Read the model definition and answer for the solid it produces. Units are mm, in the model's axes. Face numbers are marked on the shaded views. A direction names the side the tool comes from. Coordinates: 2 decimals unless noted, no trailing zeros. Write each loop counter-clockwise with the first axis right and the second up, starting at its lowest first coordinate (ties: lowest second). Pieces come first, ordered by that corner, then holes. Notation, with made-up numbers: (86.5, 82.5) -> (122.5, 82.5) arc R13 ccw to (122.5, 93.5) -> close; hole circle Ø9 at (36.25, 20). An arc over 180 degrees is marked (long way). Answer as a JSON object with one key per item and string values. Group by question number.
(1) Find section D-D (z = 27). Give the vertices of the cut face in (x, y), then the cut area to 3 significant figures.
(2) For a pull along Z with two mould halves and no side action, classify the marked faces 5, 6, 7 and 8 as +Z half, -Z half, draft (parallel to the pull), parting line (faces both ways), or undercut.
(3) Find section C-C (y = -2.27). Give the vertices of the cut face in (x, z), then the cut area to 3 significant figures.
(4) Which of the six approach directions +Z, -Z, +X, -X, +Y, -Y give full straight-line access (tool end or side, diameter ignored) to the marked faces 1, 2, 3 and 4?
(5) Straight lines are drawn through the part: L1, parallel to Z at x = -0.75, y = -0.35; L2, parallel to X at y = -0.45, z = 20.25; L3, parallel to Z at x = -8.75, y = -1.3. For each, find the intervals that lie inside material, in ascending order.
(6) Find section B-B (y = -4.2). Give the vertices of the cut face in (x, z).
(7) Flat-ended cylindrical pins translate along their axes: P1, Ø1.4, axis at x = -11, z = 18, coming from the +Y side; P2, Ø0.5, axis at x = -2.5, z = 18, coming from the +Y side; P3, Ø1, axis at y = -1.5, z = 20.5, coming from the +X side. Find the tip coordinate at first contact, or state that the pin passes through.
(8) Find section A-A (z = 24). Give the vertices of the cut face in (x, y).
from build123d import *

# Parameters (mm, degrees)
F0_W      = 15.96
F0_H      = 7.98
F1_DEPTH  = 2.94
F2_R      = 2.45
F3_DEPTH  = 1.84
F4_T      = -1.56
F5_R      = 1.535
F5_R_2    = 0.765
F6_DEPTH  = 1
F8_DEPTH  = 1.67
F10_DEPTH = 2.4
F12_DEPTH = 2.4
F13_R     = 1.555
F14_DEPTH = 10.28
F15_R     = 1.555
F16_DEPTH = 3.51


with BuildPart() as f1:
    # F0 (on Front) → F1 (new body)
    with BuildSketch(Plane.XZ):
        with Locations((-6.8829571828, 18.429612627)):
            Rectangle(F0_W, F0_H)
    extrude(amount=F1_DEPTH)

    # F2 (on face) → F3 (join)
    with BuildSketch(Plane.XZ.offset(2.94)):
        with Locations((-10.8579571828, 18.429612627)):
            Circle(F2_R)
        with Locations((-2.9079571828, 18.429612627)):
            Circle(F2_R)
    extrude(amount=F3_DEPTH)

    # F4
    f4_openings = [f1.faces().sort_by_distance(p)[0] for p in [
        (-6.882957, 0, 18.429613),
    ]]
    offset(amount=F4_T, openings=f4_openings, kind=Kind.INTERSECTION)

    # F5 (on face) → F6 (join)
    with BuildSketch(Plane(origin=(0, -1.38, 0), x_dir=(-1, 0, 0), z_dir=(0, 1, 0))):
        with Locations((6.8729571828, 18.414612627)):
            Circle(F5_R)
        with Locations((6.8729571828, 18.414612627)):
            Circle(F5_R_2, mode=Mode.SUBTRACT)
    extrude(amount=F6_DEPTH)

    # F7 (on face) → F8 (join)
    with BuildSketch(Plane.XY.offset(22.419612627)):
        Polygon((-9.0679571828, -2.94), (-9.0679571828, -1.47), (-9.0679571828, 0), (-11.4679571828, 0), (-11.4679571828, -2.94), align=None)
        Polygon((-4.6979571828, 0), (-4.6979571828, -1.47), (-4.6979571828, -2.94), (-2.2979571828, -2.94), (-2.2979571828, 0), align=None)
    extrude(amount=F8_DEPTH)

    # F9 (on face) → F10 (join)
    with BuildSketch(Plane.YZ.offset(-2.2979571828)):
        with BuildLine():
            Line((-2.27, 24.089612627), (0, 24.089612627))
            Line((0, 24.089612627), (0, 26.359612627))
            ThreePointArc((0, 26.359612627), (-0.6648676067, 24.7544802337), (-2.27, 24.089612627))
        make_face()
        with BuildLine():
            ThreePointArc((-2.94, 24.1907419532), (-2.6087946061, 24.115037341), (-2.27, 24.089612627))
            ThreePointArc((-2.27, 24.089612627), (-0.6648676067, 24.7544802337), (0, 26.359612627))
            ThreePointArc((0, 26.359612627), (-3.6175904422, 28.1863309961), (-2.94, 24.1907419532))
        make_face()
        with BuildLine():
            ThreePointArc((-0.715, 26.359612627), (-1.1704489553, 25.2600615823), (-2.27, 24.804612627))
            ThreePointArc((-2.27, 24.804612627), (-3.3695510447, 27.4591636718), (-0.715, 26.359612627))
        make_face(mode=Mode.SUBTRACT)
        with BuildLine():
            Line((-2.94, 24.089612627), (-2.27, 24.089612627))
            ThreePointArc((-2.27, 24.089612627), (-2.6087946061, 24.115037341), (-2.94, 24.1907419532))
            Line((-2.94, 24.1907419532), (-2.94, 24.089612627))
        make_face()
    extrude(amount=-F10_DEPTH)

    # F11 (on face) → F12 (join)
    with BuildSketch(Plane(origin=(-11.4679571828, 0, 0), x_dir=(0, -1, 0), z_dir=(-1, 0, 0))):
        with BuildLine():
            ThreePointArc((0, 26.359612627), (0.6648676067, 24.7544802337), (2.27, 24.089612627))
            ThreePointArc((2.27, 24.089612627), (2.6087946061, 24.115037341), (2.94, 24.1907419532))
            ThreePointArc((2.94, 24.1907419532), (4.0967183691, 25.0120221848), (4.54, 26.359612627))
            ThreePointArc((4.54, 26.359612627), (2.27, 28.629612627), (0, 26.359612627))
        make_face()
        with BuildLine():
            ThreePointArc((2.94, 24.1907419532), (2.6087946061, 24.115037341), (2.27, 24.089612627))
            Line((2.27, 24.089612627), (2.94, 24.089612627))
            Line((2.94, 24.089612627), (2.94, 24.1907419532))
        make_face()
        with BuildLine():
            Line((0, 26.359612627), (0, 24.089612627))
            Line((0, 24.089612627), (2.27, 24.089612627))
            ThreePointArc((2.27, 24.089612627), (0.6648676067, 24.7544802337), (0, 26.359612627))
        make_face()
    extrude(amount=-F12_DEPTH)

    # F13 (on face) → F14 (join)
    with BuildSketch(Plane.YZ.offset(-9.0679571828)):
        with Locations((-2.27, 26.359612627)):
            Circle(F13_R)
    extrude(amount=F14_DEPTH)

    # F15 (on face) → F16 (join)
    with BuildSketch(Plane(origin=(-11.4679571828, 0, 0), x_dir=(0, -1, 0), z_dir=(-1, 0, 0))):
        with Locations((2.27, 26.359612627)):
            Circle(F15_R)
    extrude(amount=F16_DEPTH)


solid = f1.part
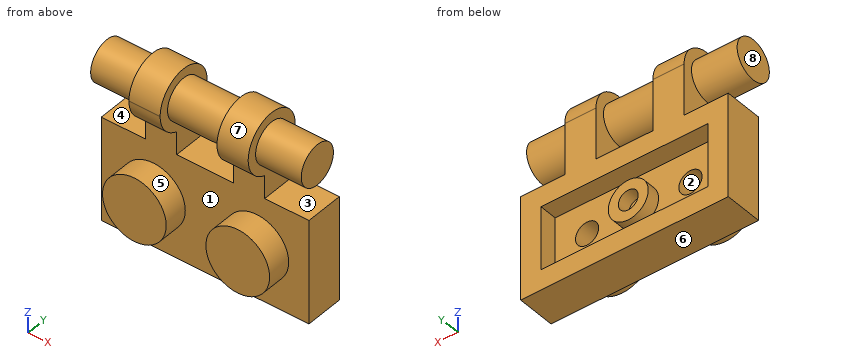
Results below:
{
 "1": {"outline": "(-14.98, -3.69) -> (-11.47, -3.69) -> (-11.47, -4.45) -> (-9.07, -4.45) -> (-9.07, -3.69) -> (-4.7, -3.69) -> (-4.7, -4.45) -> (-2.3, -4.45) -> (-2.3, -3.69) -> (1.21, -3.69) -> (1.21, -0.85) -> (-2.3, -0.85) -> (-2.3, -0.09) -> (-4.7, -0.09) -> (-4.7, -0.85) -> (-9.07, -0.85) -> (-9.07, -0.09) -> (-11.47, -0.09) -> (-11.47, -0.85) -> (-14.98, -0.85) -> close", "area": "53.2 mm2"},
 "2": {"face 5": "undercut", "face 6": "-Z half", "face 7": "undercut", "face 8": "draft"},
 "3": {"outline": "(-14.98, 24.8) -> (-11.47, 24.8) -> (-11.47, 22.42) -> (-14.86, 22.42) -> (-14.86, 14.44) -> (1.1, 14.44) -> (1.1, 22.42) -> (-2.3, 22.42) -> (-2.3, 24.8) -> (1.21, 24.8) -> (1.21, 27.91) -> (-2.3, 27.91) -> (-2.3, 28.63) -> (-4.7, 28.63) -> (-4.7, 27.91) -> (-9.07, 27.91) -> (-9.07, 28.63) -> (-11.47, 28.63) -> (-11.47, 27.91) -> (-14.98, 27.91) -> close; hole circle Ø1.78 at (-10.86, 18.43); hole (-9.07, 22.42) -> (-4.7, 22.42) -> (-4.7, 24.8) -> (-9.07, 24.8) -> close; hole circle Ø1.78 at (-2.91, 18.43)", "area": "188 mm2"},
 "4": {"face 1": "-Y", "face 2": "+Y", "face 3": "+X, +Y, -Y", "face 4": "-X, +Y, -Y"},
 "5": {"L1": "z = 14.44 to 16, 20.86 to 22.42", "L2": "x = -14.86 to -13.3, -0.46 to 1.1", "L3": "z = 14.44 to 16, 20.86 to 22.42, 25.14 to 27.57"},
 "6": {"outline": "circle Ø4.9 at (-10.86, 18.43); (-11.47, 25.16) -> (-9.07, 25.16) -> (-9.07, 27.55) -> (-11.47, 27.55) -> close; circle Ø4.9 at (-2.91, 18.43); (-4.7, 25.16) -> (-2.3, 25.16) -> (-2.3, 27.55) -> (-4.7, 27.55) -> close"},
 "7": {"P1": "stops at y = -1.38", "P2": "stops at y = -3.22", "P3": "stops at x = 1.1"},
 "8": {"outline": "(-11.47, -2.94) -> (-9.07, -2.94) -> (-9.07, 0) -> (-11.47, 0) -> close; (-4.7, -2.94) -> (-2.3, -2.94) -> (-2.3, 0) -> (-4.7, 0) -> close"}
}
